The listing builds one solid part. Answer for the finished solid, in the listing's coordinates (mm). Face numbers are marked on the shaded views. A direction names the side the tool comes from. Coordinates: 2 decimals unless noted, no trailing zeros. Write each loop counter-clockwise with the first axis right and the second up, starting at its lowest first coordinate (ties: lowest second). Pieces come first, ordered by that corner, then holes.
(1) The part is cut by section B-B on x = 1.75. Determine the outline of the cut face in (y, z), plus the area to 3 significant figures.
(2) Straight lines are drawn through the part: line 1 (X direction, y = 6.95, z = -5.2); line 2 (Y direction, x = 4.25, z = -2.25); line 3 (Y direction, x = 9.5, z = -5.25). For each, find the intervals that lie inside material, in ascending order.
(3) The part is cut by section A-A on y = 7. Determine the outline of the cut face in (x, z).
(4) The part is cut by section D-D on x = 3.5. Determine the outline of the cut face in (y, z), plus the area to 3 significant figures.
(5) Given P1, Ø1, axis at x = 8.5, z = -5.5, coming from the +Y side, flat-ended and moving along its own axis, determine where the tip first touches the part or whether it passes through.
(6) Which of the six approach directions +Z, -Z, +X, -X, +Y, -Y give full straight-line access (tool end or side, diameter ignored) to the marked faces 4 and 5?
(7) For a pull along X with two mould halves and no side action, classify the marked faces 1, 2 and 3 as +X half, -X half, draft (parallel to the pull), parting line (faces both ways), or undercut.
(8) The part is cut by section C-C on z = -5.2. Determine the outline of the cut face in (x, y), plus the area to 3 significant figures.
from build123d import *

# Parameters (mm, degrees)
SKETCH_1_W          = 14
SKETCH_1_H          = 7.2
EXTRUDE_1_DEPTH     = 8.5
CHAMFER_1_SIZE      = 3
SKETCH_2_R          = 1
CUT_EXTRUDE_1_DEPTH = 4


with BuildPart() as part:
    # Эскиз1 → Бобышка-Вытянуть1 (new body)
    with BuildSketch(Plane(origin=(0, 0, 0), x_dir=(1, 0, 0), z_dir=(0, 1, 0))):
        with Locations((7, 3.6)):
            Rectangle(SKETCH_1_W, SKETCH_1_H)
    extrude(amount=EXTRUDE_1_DEPTH)

    # Фаска1
    chamfer_1_edges = [part.edges().sort_by_distance(p)[0] for p in [
        (7, 8.5, 0),
    ]]
    chamfer(chamfer_1_edges, length=CHAMFER_1_SIZE)

    # Эскиз2 → Вырез-Вытянуть1 (cut)
    with BuildSketch(Plane(origin=(0, 8.5, 0), x_dir=(1, 0, 0), z_dir=(0, 1, 0))):
        with Locations(Location((1.75, 5.2, 0), (0, 0, 270))):
            Circle(SKETCH_2_R)
        with Locations(Location((5.25, 5.2, 0), (0, 0, 270))):
            Circle(SKETCH_2_R)
        with Locations(Location((8.75, 5.2, 0), (0, 0, 270))):
            Circle(SKETCH_2_R)
        with Locations(Location((12.25, 5.2, 0), (0, 0, 270))):
            Circle(SKETCH_2_R)
    extrude(amount=-CUT_EXTRUDE_1_DEPTH, mode=Mode.SUBTRACT)


solid = part.part
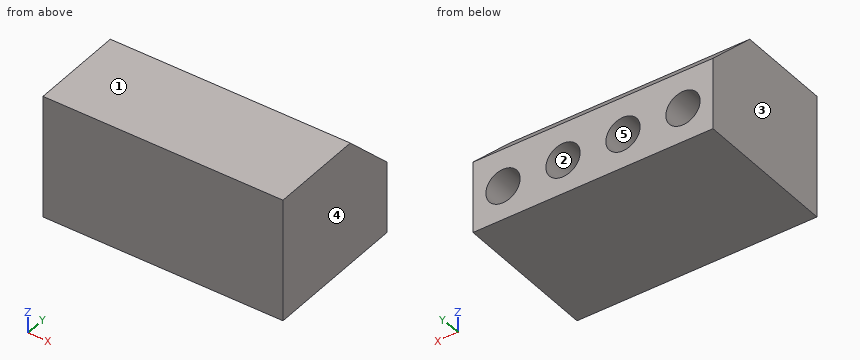
Model answer:
1. outline: (0, -7.2) - (8.5, -7.2) - (8.5, -6.2) - (4.5, -6.2) - (4.5, -4.2) - (8.5, -4.2) - (8.5, -3) - (5.5, 0) - (0, 0) - close
1. area: 48.7 mm2
2. line 1: x = 0 to 0.75, 2.75 to 4.25, 6.25 to 7.75, 9.75 to 11.25, 13.25 to 14
2. line 2: y = 0 to 7.75
2. line 3: y = 0 to 4.5
3. outline: (0, -7.2) - (14, -7.2) - (14, -1.5) - (0, -1.5) - close; hole circle Ø2 at (1.75, -5.2); hole circle Ø2 at (5.25, -5.2); hole circle Ø2 at (8.75, -5.2); hole circle Ø2 at (12.25, -5.2)
4. outline: (0, -7.2) - (8.5, -7.2) - (8.5, -3) - (5.5, 0) - (0, 0) - close
4. area: 56.7 mm2
5. P1: stops at y = 4.5
6. face 4: +Z, -Z, +X, +Y, -Y
6. face 5: +Y
7. face 1: draft
7. face 2: undercut
7. face 3: -X half
8. outline: (0, 0) - (14, 0) - (14, 8.5) - (13.25, 8.5) - (13.25, 4.5) - (11.25, 4.5) - (11.25, 8.5) - (9.75, 8.5) - (9.75, 4.5) - (7.75, 4.5) - (7.75, 8.5) - (6.25, 8.5) - (6.25, 4.5) - (4.25, 4.5) - (4.25, 8.5) - (2.75, 8.5) - (2.75, 4.5) - (0.75, 4.5) - (0.75, 8.5) - (0, 8.5) - close
8. area: 87.0 mm2
